Here's how the part is built. I have some questions about the finished solid (model axes, mm). Coordinates: 2 decimals unless noted, no trailing zeros. Loops run counter-clockwise (first coordinate to the right, second up) from the corner with the lowest first, then second, coordinate; pieces in that order, holes last. Notation, with made-up numbers: (-0.5, 59.25) - (22.5, 59.25) arc R17 ccw to (22.5, 86.25) - close; hole circle Ø7 at (-14, 47). An arc over 180 degrees is marked (long way). Use a Markdown table: item, result.
Autodesk Inventor part; units mm, degrees
ref_plane "YZ Plane" through (0, 0, 0) normal (1, 0, 0) x (0, 1, 0)
ref_plane "XZ Plane" through (0, 0, 0) normal (0, 1, 0) x (-1, 0, 0)
ref_plane "XY Plane" through (0, 0, 0) normal (0, 0, 1) x (1, 0, 0)
sketch "Sketch_1" plane through (0, 0, 0) normal (0, 0, 1) x (1, 0, 0)
  line L0 (7, 0) -> (0, 0)
  line L1 (0, 9) -> (0, 5.25)
  line L2 (0, 5.25) -> (0.25, 5)
  line L3 (0.25, 5) -> (7, 5)
  line L4 (7, 5) -> (7, 5.75)
  line L5 (7, 5.75) -> (6.75, 6)
  line L6 (6.75, 6) -> (1, 6)
  line L7 (1, 6) -> (1, 9)
  line L8 (1, 9) -> (0, 9)
revolve "Revolution1" add sketch "Sketch_1" angle 360 about axis through (7, 0, 0) along (1, 0, 0)
properties part number "SKF_PPMF 101207"
Q1. I want a section at C-C, the plane x = 2.25. Write out the boundary of the cut face in (y, z), then the cut area to 3 significant figures.
Check values:
| item | result |
|---|---|
| outline | circle Ø12 at (0, 0); hole circle Ø10 at (0, 0) |
| area | 34.6 mm^2 |
Q2. I want a section at A-A, the plane z = 0. Write out the boundary of the cut face in (x, y), then the cut area to 3 significant figures.
Check values:
| item | result |
|---|---|
| outline | (0, -9) - (1, -9) - (1, -6) - (6.75, -6) - (7, -5.75) - (7, -5) - (0.25, -5) - (0, -5.25) - close; (0, 5.25) - (0.25, 5) - (7, 5) - (7, 5.75) - (6.75, 6) - (1, 6) - (1, 9) - (0, 9) - close |
| area | 19.9 mm^2 |
Q3. If we mould it in two halves opening along Y, with no side actions, what happens to faces 1 (the face through (4, -6, 0)), 2 (the face through (1, 2, -6)), 3 (the face through (3.67, -1.08, -4.88))? For each: pulls with the +Y half, pulls with the -Y half, needs draft (parallel to the pull), parting line crosses it, or undercut.
Check values:
| item | result |
|---|---|
| face 1 | parting line crosses it |
| face 2 | needs draft |
| face 3 | undercut |
Q4. Will these pins go through, and if not, where does the flat tip stop? P1, Ø1, axis at y = 1, z = 7, coming from the +X side; P2, Ø1.5, axis at x = 3, y = -0.5, coming from the -Z side.
Check values:
| item | result |
|---|---|
| P1 | x = 1 |
| P2 | z = -6 |
Q5. I want a section at D-D, the plane z = 6.5. Write out the boundary of the cut face in (x, y), then the cut area to 3 significant figures.
Check values:
| item | result |
|---|---|
| outline | (0, -6.22) - (1, -6.22) - (1, 6.22) - (0, 6.22) - close |
| area | 12.4 mm^2 |
Q6. Please list where these lines run through material, in increasing order: L1, parallel to Z at x = 1.75, y = 0; L2, parallel to X at y = -3.25, z = -7; L3, parallel to Z at x = 3, y = 2.75. Write a range as from..to.
Check values:
| item | result |
|---|---|
| L1 | -6..-5, 5..6 |
| L2 | 0..1 |
| L3 | -5.33..-4.18, 4.18..5.33 |
